Here's how the part is built. I have some questions about the finished solid (model axes, mm). Face numbers are marked on the shaded views. A direction names the side the tool comes from. Give positions to 0.01 mm unless a question says otherwise; leave off trailing zeros. Loops run counter-clockwise (first coordinate to the right, second up) from the corner with the lowest first, then second, coordinate; pieces in that order, holes last. Notation, with made-up numbers: (-38.75, -18.75) - (-19.75, -18.75) arc R15 cw to (-19.75, -10.75) - close; hole circle Ø7 at (-27.5, 49.5). An arc over 180 degrees is marked (long way). Use one line per item in the form item = value.
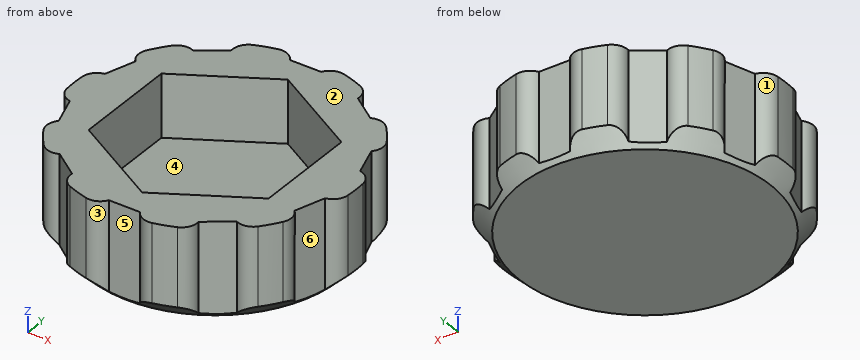
from build123d import *

# Parameters (mm, degrees)
F0_R        = 9
F1_DEPTH    = 4
F2_R        = 9
F3_DEPTH    = 2
F4_SIZE     = 1
F5_W        = 2
F5_H        = 1.5
F6_DEPTH    = 6.001
F7_T1_DEPTH = 10.6633310907


# Not quite as in the source:
# - a fillet or chamfer that OpenCascade refuses, or shapes differently, is made with other operations: its cross-section is extruded or revolved along the edge and cut away or added


with BuildPart() as f1:
    # F0 (on Top) → F1 (new body)
    with BuildSketch(Plane.XY):
        Circle(F0_R)
        Polygon((-5.75, 3.3197640478), (0, 6.6395280957), (5.75, 3.3197640478), (5.75, -3.3197640478), (0, -6.6395280957), (-5.75, -3.3197640478), align=None, mode=Mode.SUBTRACT)
    extrude(amount=F1_DEPTH)

    # F2 (on face) → F3 (join)
    with BuildSketch(Plane(origin=(0, 0, 0), x_dir=(1, 0, 0), z_dir=(0, 0, -1))):
        Circle(F2_R)
    extrude(amount=F3_DEPTH)

    # F4
    f4_edges = [f1.edges().sort_by_distance(p)[0] for p in [
        (-9, 0, -2),
    ]]
    chamfer(f4_edges, length=F4_SIZE)

    # F5 (on face) → F6 (cut, through all)
    with BuildSketch(Plane.XY.offset(4)):
        with Locations((0, 9)):
            Rectangle(F5_W, F5_H)
        Polygon((-4.040211337, 7.2621754559), (-4.9218892155, 8.4757009474), (-6.5399232042, 7.3001304429), (-5.6582453258, 6.0866049513), align=None)
        Polygon((-7.5371992651, 3.5004467199), (-8.9637840395, 3.9639722115), (-9.5818180283, 2.0618591789), (-8.1552332538, 1.5983336873), align=None)
        Polygon((-8.1552332538, -1.5983336873), (-9.5818180283, -2.0618591789), (-8.9637840395, -3.9639722115), (-7.5371992651, -3.5004467199), align=None)
        Polygon((-5.6582453258, -6.0866049513), (-6.5399232042, -7.3001304429), (-4.9218892155, -8.4757009474), (-4.040211337, -7.2621754559), align=None)
        with Locations((0, -9)):
            Rectangle(F5_W, F5_H)
        Polygon((4.040211337, -7.2621754559), (4.9218892155, -8.4757009474), (6.5399232042, -7.3001304429), (5.6582453258, -6.0866049513), align=None)
        Polygon((7.5371992651, -3.5004467199), (8.9637840395, -3.9639722115), (9.5818180283, -2.0618591789), (8.1552332538, -1.5983336873), align=None)
        Polygon((8.1552332538, 1.5983336873), (9.5818180283, 2.0618591789), (8.9637840395, 3.9639722115), (7.5371992651, 3.5004467199), align=None)
        Polygon((5.6582453258, 6.0866049513), (6.5399232042, 7.3001304429), (4.9218892155, 8.4757009474), (4.040211337, 7.2621754559), align=None)
    extrude(amount=-F6_DEPTH, mode=Mode.SUBTRACT)

    # F7: fillet of radius 1 on 20 edges, made by hand

    # F7_s2 → F7_t1 (cut)
    with BuildSketch(Plane.XY.offset(-3.8316655453)):
        with BuildLine():
            ThreePointArc((2.1155025829, 8.7478368081), (1.4729019887, 8.6890401766), (1, 8.25))
            Line((1, 8.25), (1, 8.94427191))
            ThreePointArc((1, 8.94427191), (1.5608445705, 8.8636202664), (2.1155025829, 8.7478368081))
        make_face()
        with BuildLine():
            ThreePointArc((4.040211337, 7.2621754559), (3.9156869325, 7.8953312347), (3.4303719241, 8.3206098612))
            ThreePointArc((3.4303719241, 8.3206098612), (3.9471554914, 8.0882608469), (4.4482941268, 7.8238532298))
            Line((4.4482941268, 7.8238532298), (4.040211337, 7.2621754559))
        make_face()
        with BuildLine():
            ThreePointArc((6.8533270065, 5.8336874224), (6.2988924123, 6.1638311007), (5.6582453258, 6.0866049513))
            Line((5.6582453258, 6.0866049513), (6.0663281156, 6.6482827252))
            ThreePointArc((6.0663281156, 6.6482827252), (6.4726550576, 6.2533780075), (6.8533270065, 5.8336874224))
        make_face()
        with BuildLine():
            ThreePointArc((7.5371992651, 3.5004467199), (7.8086165348, 4.0858741136), (7.6659609501, 4.7151927544))
            ThreePointArc((7.6659609501, 4.7151927544), (7.9474763144, 4.2234606937), (8.1974910891, 3.7149885388))
            Line((8.1974910891, 3.7149885388), (7.5371992651, 3.5004467199))
        make_face()
        with BuildLine():
            ThreePointArc((8.9734134496, 0.691267721), (8.7189200259, 1.2842480452), (8.1552332538, 1.5983336873))
            Line((8.1552332538, 1.5983336873), (8.8155250779, 1.8128755062))
            ThreePointArc((8.8155250779, 1.8128755062), (8.9121313102, 1.2545578943), (8.9734134496, 0.691267721))
        make_face()
        with BuildLine():
            ThreePointArc((8.9734134496, -0.691267721), (8.7189200259, -1.2842480452), (8.1552332538, -1.5983336873))
            Line((8.1552332538, -1.5983336873), (8.8155250779, -1.8128755062))
            ThreePointArc((8.8155250779, -1.8128755062), (8.9121313102, -1.2545578943), (8.9734134496, -0.691267721))
        make_face()
        with BuildLine():
            ThreePointArc((7.6659609501, -4.7151927544), (7.8086165348, -4.0858741136), (7.5371992651, -3.5004467199))
            Line((7.5371992651, -3.5004467199), (8.1974910891, -3.7149885388))
            ThreePointArc((8.1974910891, -3.7149885388), (7.9474763144, -4.2234606937), (7.6659609501, -4.7151927544))
        make_face()
        with BuildLine():
            ThreePointArc((5.6582453258, -6.0866049513), (6.2988924123, -6.1638311007), (6.8533270065, -5.8336874224))
            ThreePointArc((6.8533270065, -5.8336874224), (6.4726550576, -6.2533780075), (6.0663281156, -6.6482827252))
            Line((6.0663281156, -6.6482827252), (5.6582453258, -6.0866049513))
        make_face()
        with BuildLine():
            ThreePointArc((3.4303719241, -8.3206098612), (3.9156869325, -7.8953312347), (4.040211337, -7.2621754559))
            Line((4.040211337, -7.2621754559), (4.4482941268, -7.8238532298))
            ThreePointArc((4.4482941268, -7.8238532298), (3.9471554914, -8.0882608469), (3.4303719241, -8.3206098612))
        make_face()
        with BuildLine():
            ThreePointArc((1, -8.25), (1.4729019887, -8.6890401766), (2.1155025829, -8.7478368081))
            ThreePointArc((2.1155025829, -8.7478368081), (1.5608445705, -8.8636202664), (1, -8.94427191))
            Line((1, -8.94427191), (1, -8.25))
        make_face()
        with BuildLine():
            ThreePointArc((-2.1155025829, -8.7478368081), (-1.4729019887, -8.6890401766), (-1, -8.25))
            Line((-1, -8.25), (-1, -8.94427191))
            ThreePointArc((-1, -8.94427191), (-1.5608445705, -8.8636202664), (-2.1155025829, -8.7478368081))
        make_face()
        with BuildLine():
            ThreePointArc((-4.040211337, -7.2621754559), (-3.9156869325, -7.8953312347), (-3.4303719241, -8.3206098612))
            ThreePointArc((-3.4303719241, -8.3206098612), (-3.9471554914, -8.0882608469), (-4.4482941268, -7.8238532298))
            Line((-4.4482941268, -7.8238532298), (-4.040211337, -7.2621754559))
        make_face()
        with BuildLine():
            ThreePointArc((-6.8533270065, -5.8336874224), (-6.2988924123, -6.1638311007), (-5.6582453258, -6.0866049513))
            Line((-5.6582453258, -6.0866049513), (-6.0663281156, -6.6482827252))
            ThreePointArc((-6.0663281156, -6.6482827252), (-6.4726550576, -6.2533780075), (-6.8533270065, -5.8336874224))
        make_face()
        with BuildLine():
            ThreePointArc((-7.5371992651, -3.5004467199), (-7.8086165348, -4.0858741136), (-7.6659609501, -4.7151927544))
            ThreePointArc((-7.6659609501, -4.7151927544), (-7.9474763144, -4.2234606937), (-8.1974910891, -3.7149885388))
            Line((-8.1974910891, -3.7149885388), (-7.5371992651, -3.5004467199))
        make_face()
        with BuildLine():
            ThreePointArc((-8.9734134496, -0.691267721), (-8.7189200259, -1.2842480452), (-8.1552332538, -1.5983336873))
            Line((-8.1552332538, -1.5983336873), (-8.8155250779, -1.8128755062))
            ThreePointArc((-8.8155250779, -1.8128755062), (-8.9121313102, -1.2545578943), (-8.9734134496, -0.691267721))
        make_face()
        with BuildLine():
            ThreePointArc((-8.1552332538, 1.5983336873), (-8.7189200259, 1.2842480452), (-8.9734134496, 0.691267721))
            ThreePointArc((-8.9734134496, 0.691267721), (-8.9121313102, 1.2545578943), (-8.8155250779, 1.8128755062))
            Line((-8.8155250779, 1.8128755062), (-8.1552332538, 1.5983336873))
        make_face()
        with BuildLine():
            ThreePointArc((-7.6659609501, 4.7151927544), (-7.8086165348, 4.0858741136), (-7.5371992651, 3.5004467199))
            Line((-7.5371992651, 3.5004467199), (-8.1974910891, 3.7149885388))
            ThreePointArc((-8.1974910891, 3.7149885388), (-7.9474763144, 4.2234606937), (-7.6659609501, 4.7151927544))
        make_face()
        with BuildLine():
            ThreePointArc((-5.6582453258, 6.0866049513), (-6.2988924123, 6.1638311007), (-6.8533270065, 5.8336874224))
            ThreePointArc((-6.8533270065, 5.8336874224), (-6.4726550576, 6.2533780075), (-6.0663281156, 6.6482827252))
            Line((-6.0663281156, 6.6482827252), (-5.6582453258, 6.0866049513))
        make_face()
        with BuildLine():
            ThreePointArc((-3.4303719241, 8.3206098612), (-3.9156869325, 7.8953312347), (-4.040211337, 7.2621754559))
            Line((-4.040211337, 7.2621754559), (-4.4482941268, 7.8238532298))
            ThreePointArc((-4.4482941268, 7.8238532298), (-3.9471554914, 8.0882608469), (-3.4303719241, 8.3206098612))
        make_face()
        with BuildLine():
            ThreePointArc((-1, 8.25), (-1.4729019887, 8.6890401766), (-2.1155025829, 8.7478368081))
            ThreePointArc((-2.1155025829, 8.7478368081), (-1.5608445705, 8.8636202664), (-1, 8.94427191))
            Line((-1, 8.94427191), (-1, 8.25))
        make_face()
    extrude(amount=F7_T1_DEPTH, mode=Mode.SUBTRACT)


solid = f1.part
(1) For the marked faces 4, 5 and 6, which set-ups out of +Z, -Z, +X, -X, +Y, -Y let a thin tool reach every point of the face, with its end or its side?
Geometry says:
face_4 = +Z
face_5 = +Z, -Z, -Y
face_6 = +Z, -Z, +X
(2) If I drill on probe 1 along X at (y, z) = (0.25, 3); probe 2 along Z at (x, y) = (-3, 3.5); probe 3 along X at (y, z) = (-6.25, 1.25), over which ranges is the centre line in solid material (lowest first)?
Geometry says:
probe_1 = -9 to -5.75, 5.75 to 9
probe_2 = -2 to 0
probe_3 = -5.43 to -0.67, 0.67 to 5.43
(3) For P1, Ø2, axis at x = 0.5, z = 2.5, coming from the +Y side; P2, Ø1.5, axis at y = -2.5, z = 0.5, coming from the -X side; P3, Ø1.6, axis at x = 0, z = 1, coming from the -Y side, each with a flat end and sliding along its axis, tell me the tip position at first contact or that it passes through.
Geometry says:
P1 = 8.7
P2 = -8.11
P3 = -8.25
(4) If we section it at A-A (y = 0): List the corners of the cut face in (x, z) for me, plus the area to 3 significant figures.
Geometry says:
outline = (-9, -1) - (-8, -2) - (8, -2) - (9, -1) - (9, 4) - (5.75, 4) - (5.75, 0) - (-5.75, 0) - (-5.75, 4) - (-9, 4) - close
area = 61.0 mm²
(5) Thinking about a two-plate mould opening in X: for the marked faces 1, 2 and 3, which applies, pulls with the +X half, pulls with the -X half, needs draft (parallel to the pull), parting line crosses it, or undercut?
Geometry says:
face_1 = pulls with the -X half
face_2 = needs draft
face_3 = undercut
